from build123d import *

# Parameters (mm, degrees)
F0_R     = 4
F1_DEPTH = 6
F3_DEPTH = 35
F5_DEPTH = 45


with BuildPart() as f1:
    # F0 (on Top) → F1 (new body)
    with BuildSketch(Plane.XY):
        Polygon((20, -15), (60, -15), (60, 15), (0, 15), (-20, 15), (-60, 15), (-60, -15), (0, -15), align=None)
        with Locations((-40, 0)):
            Circle(F0_R, mode=Mode.SUBTRACT)
        with Locations((40, 0)):
            Circle(F0_R, mode=Mode.SUBTRACT)
    extrude(amount=F1_DEPTH)

    # F2 (on face) → F3 (join)
    with BuildSketch(Plane.XY.offset(6)):
        Polygon((20, 15), (0, 15), (-20, 15), (-20, -15), (20, -15), align=None)
    extrude(amount=F3_DEPTH)

    # F4 (on face) → F5 (cut)
    with BuildSketch(Plane.YZ.offset(20)):
        with BuildLine():
            Line((15, 41), (0, 41))
            ThreePointArc((0, 41), (10.606602, 36.606602), (15, 26))
            Line((15, 26), (15, 41))
        make_face()
        with BuildLine():
            ThreePointArc((-15, 26), (-10.606602, 36.606602), (0, 41))
            Line((0, 41), (-15, 41))
            Line((-15, 41), (-15, 26))
        make_face()
        with BuildLine():
            ThreePointArc((4, 26), (2.828427, 28.828427), (0, 30))
            ThreePointArc((0, 30), (-2.828427, 23.171573), (4, 26))
        make_face()
    extrude(amount=-F5_DEPTH, mode=Mode.SUBTRACT)


solid = f1.part
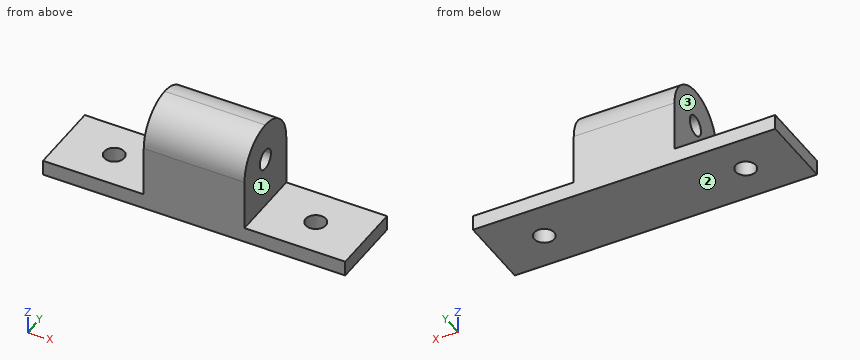
Here's how the part is built. I have some questions about the finished solid (model axes, mm). Face numbers are marked on the shaded views. A direction names the side the tool comes from. Round coordinates to 2 decimals unless told otherwise and drop trailing zeros. Loops run counter-clockwise (first coordinate to the right, second up) from the corner with the lowest first, then second, coordinate; pieces in that order, holes last. Notation, with made-up numbers: M 74.25,49.5 L 93.25,49.5 A29 ccw 93.25,76.5 Z; hole C 41,-17 d7. An arc over 180 degrees is marked long. Write each question's results on one line, items separated by ' | '. Start each with the question number.
(1) I want a section at C-C (y = -8.5). Please give me the cut outline in (x, z).
(2) Will these pins go through, and if not, where does the flat tip stop? P1, Ø5, axis at x = -36, y = 3.5, coming from the +Z side; P2, Ø8, axis at x = -36.5, z = 11.5, coming from the +Y side; P3, Ø15, axis at y = 2.5, z = 30.5, coming from the +X side; P4, Ø5, axis at x = -16, y = -3, coming from the +Z side.
(3) On a 3-axis mill with a long thin cutter (end or side, diameter ignored), from which of +Z, -Z, +X, -X, +Y, -Y can I reach the whole of each face in a straight line? I mean the marked faces 1, 2 and 3. Say none if no direction works.
(4) I want a section at B-B (y = 2). Please give me the cut outline in (x, z).
(5) If I drill on probe 1 along Y at (x, z) = (40, 1); probe 2 along Z at (x, y) = (1, 0); probe 3 along Z at (x, y) = (40.5, -5.5), over which ranges is the centre line in solid material (lowest first)? Write a range as from..to.
(6) I want a section at D-D (z = 13). Please give me the cut outline in (x, y).
(7) I want a section at A-A (x = -40). Please give me the cut outline in (y, z).
Solved:
1) outline: M -60,0 L 60,0 L 60,6 L 20,6 L 20,38.36 L -20,38.36 L -20,6 L -60,6 Z
2) P1: stops at z = 6 | P2: passes through | P3: stops at x = 20 | P4: stops at z = 40.99
3) face 1: +Z, +X, +Y, -Y | face 2: -Z, +X, -X, +Y, -Y | face 3: +Z, -X, +Y, -Y
4) outline: M -60,0 L -43.46,0 L -43.46,6 L -60,6 Z; M -36.54,0 L 36.54,0 L 36.54,6 L 20,6 L 20,22.54 L -20,22.54 L -20,6 L -36.54,6 Z; M -20,29.46 L 20,29.46 L 20,40.87 L -20,40.87 Z; M 43.46,0 L 60,0 L 60,6 L 43.46,6 Z
5) probe 1: y = -15..-4, 4..15 | probe 2: z = 0..22, 30..41 | probe 3: z = 0..6
6) outline: M -20,-15 L 20,-15 L 20,15 L -20,15 Z
7) outline: M -15,0 L -4,0 L -4,6 L -15,6 Z; M 4,0 L 15,0 L 15,6 L 4,6 Z
